Source: CAD feature listing. Evaluate the final solid. Frame: model axes, mm. Give positions to 0.01 mm unless a question says otherwise; leave off trailing zeros. Loops run counter-clockwise (first coordinate to the right, second up) from the corner with the lowest first, then second, coordinate; pieces in that order, holes last. Notation, with made-up numbers: (66, 62) -> (85, 62) arc R30 ccw to (85, 98) -> close; hole circle Ø2 at (9, 53.25). An arc over 180 degrees is marked (long way). Return JSON: item names as keys, results as strings. Group by question number.
(1) Pin query (flat end, axial travel): pin 1 (4 mm diameter, centred on x = -8.5, z = -3, fed in from +Y). Return the tip coordinate at first contact, or that it passes through.
(2) Cut plane C-C on y = 2.5. Return loops of the section in (x, z), then the cut area to 3 significant figures.
(3) Ray query, line 1 (X direction, y = 1.25, z = -15.5); line 2 (X direction, y = 1.4, z = 0). Return the intervals inside material, ascending. Write a range as from..to.
(4) Cut plane D-D on z = 0. Return loops of the section in (x, y).
(5) Cut plane A-A on x = -15.5. Return loops of the section in (y, z).
(6) Cut plane B-B on z = 15.5. Return loops of the section in (x, y), then the cut area to 3 significant figures.
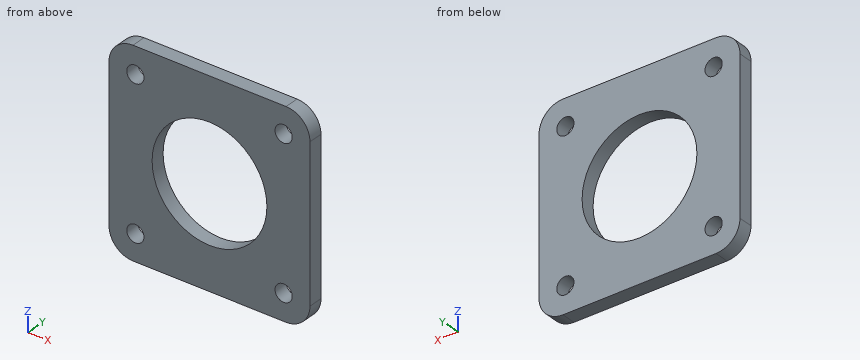
```python
from build123d import *

# Parameters (mm, degrees)
SKETCH1_W            = 42
SKETCH1_H            = 42
BOSS_EXTRUDE1_DEPTH  = 3
M3_CLEARANCE_HOLE1_D = 3.6
SKETCH4_R            = 12
CUT_EXTRUDE1_DEPTH   = 4
FILLET1_R            = 5


with BuildPart() as part:
    # Sketch1 → Boss-Extrude1 (new body)
    with BuildSketch(Plane(origin=(0, 0, 0), x_dir=(1, 0, 0), z_dir=(0, 1, 0))):
        Rectangle(SKETCH1_W, SKETCH1_H)
    extrude(amount=BOSS_EXTRUDE1_DEPTH)

    # M3 Clearance Hole1 (through all)
    with Locations(Plane(origin=(0, 3, 0), x_dir=(1, 0, 0), z_dir=(0, 1, 0))):
        with Locations((-15.5, 15.5), (-15.5, -15.5), (15.5, -15.5), (15.5, 15.5)):
            Hole(M3_CLEARANCE_HOLE1_D / 2)

    # Sketch4 → Cut-Extrude1 (cut, through all)
    with BuildSketch(Plane(origin=(0, 3, 0), x_dir=(1, 0, 0), z_dir=(0, 1, 0))):
        Circle(SKETCH4_R)
    extrude(amount=-CUT_EXTRUDE1_DEPTH, mode=Mode.SUBTRACT)

    # Fillet1
    fillet1_edges = [part.edges().sort_by_distance(p)[0] for p in [
        (-21, 1.5, -21),
        (21, 1.5, -21),
        (21, 1.5, 21),
        (-21, 1.5, 21),
    ]]
    fillet(fillet1_edges, radius=FILLET1_R)


solid = part.part
```
Answers:
{
 "1": {"pin 1": "through"},
 "2": {"outline": "(-21, -16) arc R5 ccw to (-16, -21) -> (16, -21) arc R5 ccw to (21, -16) -> (21, 16) arc R5 ccw to (16, 21) -> (-16, 21) arc R5 ccw to (-21, 16) -> close; hole circle Ø3.6 at (-15.5, -15.5); hole circle Ø3.6 at (-15.5, 15.5); hole circle Ø24 at (0, 0); hole circle Ø3.6 at (15.5, -15.5); hole circle Ø3.6 at (15.5, 15.5)", "area": "1,250 mm²"},
 "3": {"line 1": "-21..-17.3, -13.7..13.7, 17.3..21", "line 2": "-21..-12, 12..21"},
 "4": {"outline": "(-21, 0) -> (-12, 0) -> (-12, 3) -> (-21, 3) -> close; (12, 0) -> (21, 0) -> (21, 3) -> (12, 3) -> close"},
 "5": {"outline": "(0, -21) -> (3, -21) -> (3, -17.3) -> (0, -17.3) -> close; (0, -13.7) -> (3, -13.7) -> (3, 13.7) -> (0, 13.7) -> close; (0, 17.3) -> (3, 17.3) -> (3, 21) -> (0, 21) -> close"},
 "6": {"outline": "(-21, 0) -> (-17.3, 0) -> (-17.3, 3) -> (-21, 3) -> close; (-13.7, 0) -> (13.7, 0) -> (13.7, 3) -> (-13.7, 3) -> close; (17.3, 0) -> (21, 0) -> (21, 3) -> (17.3, 3) -> close", "area": "104 mm²"}
}
